Part print with two shaded views. Sizes in mm from the minimum x, y, z corner. A direction names the side the tool comes from. Coordinates: 2 decimals unless noted, no trailing zeros. Loops run counter-clockwise (first coordinate to the right, second up) from the corner with the lowest first, then second, coordinate; pieces in that order, holes last. Notation, with made-up numbers: (80.25, 83.25) -> (137.25, 83.25) arc R9 cw to (137.25, 100.25) -> close; hole circle Ø2 at (1.25, 13). An arc over 180 degrees is marked (long way). Use one line per item in the form item = value.
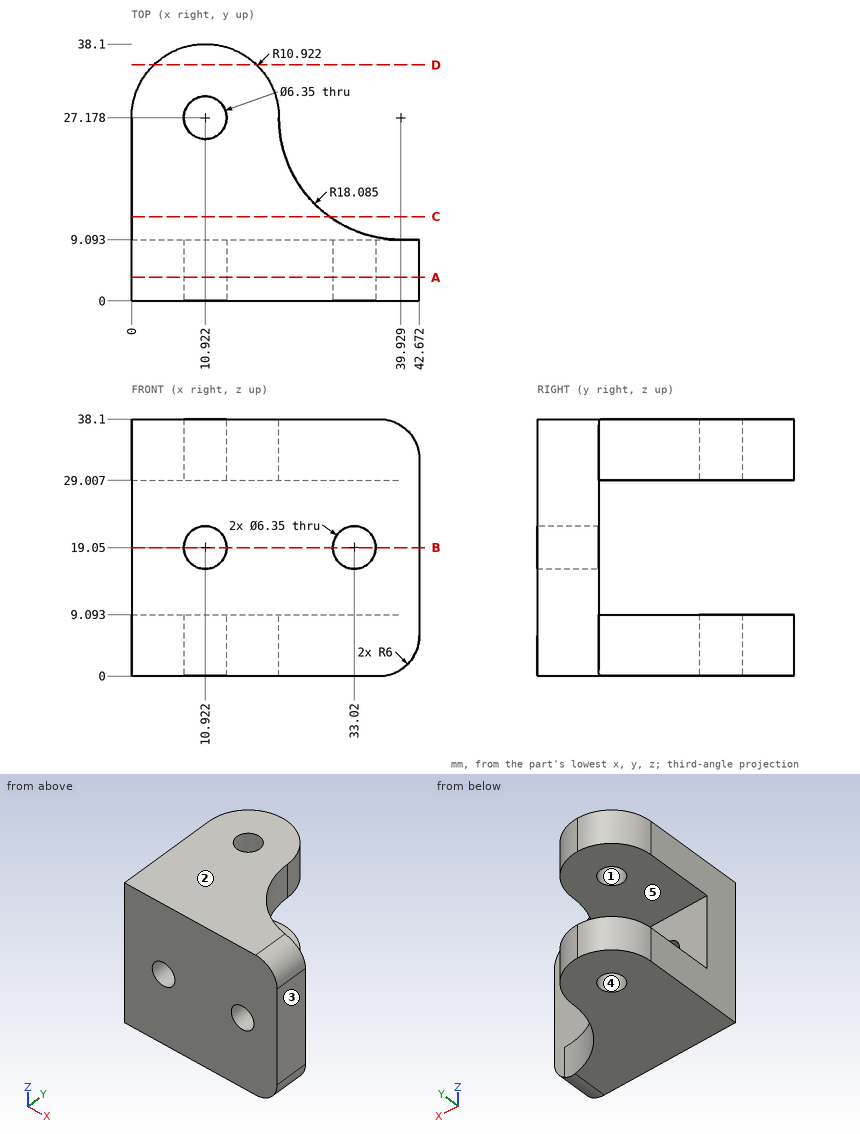
Q1. Which spindle directions (+Z, -Z, +X, -X, +Y, -Y) get a long thin tool onto all of the face, cutting with end or side? Do the marked faces 4 and 5. Say none if no direction does.
Result:
face_4 = +Z, -Z
face_5 = +X, -X, +Y
Q2. Band-saw the part on D-D, the plane y = 35. Write the cut outline in (x, z) (1 decimal), and give its area (3 significant figures).
Result:
outline = (3.3, 0) -> (18.5, 0) -> (18.5, 9.1) -> (3.3, 9.1) -> close; (3.3, 29) -> (18.5, 29) -> (18.5, 38.1) -> (3.3, 38.1) -> close
area = 277 mm2
Q3. Band-saw the part on C-C, the plane y = 12.5. Write the cut outline in (x, z), and give its area (3 significant figures).
Result:
outline = (0, 0) -> (29.36, 0) -> (29.36, 9.09) -> (0, 9.09) -> close; (0, 29.01) -> (29.36, 29.01) -> (29.36, 38.1) -> (0, 38.1) -> close
area = 534 mm2
Q4. Mould opens along X. For the marked faces 1, 2 and 3 say: released by +X, released by -X, zero draft, split by the parting line, or undercut.
Result:
face_1 = undercut
face_2 = zero draft
face_3 = released by +X
Q5. Wall check: line 1 along X through (y, z) = (5.25, 19.05) (3 decimals); line 2 along Z through (x, y) = (19.5, 31); line 3 along Y through (x, z) = (39.5, 3.5). Give the ranges that are in metal, low to high.
Result:
line_1 = 0 to 7.747, 14.097 to 29.845, 36.195 to 42.672
line_2 = 0 to 9.09, 29.01 to 38.1
line_3 = 0 to 9.1
Q6. Pin check, flat tip, straight feed: pin 1 Ø1 at (x, z) = (11, 17) entering from +Y. Stop position of the tip, or through.
Result:
pin_1 = through
Q7. Band-saw the part on B-B, the plane z = 19.05. Write the cut outline in (x, y) (1 decimal).
Result:
outline = (0, 0) -> (7.7, 0) -> (7.7, 9.1) -> (0, 9.1) -> close; (14.1, 0) -> (29.8, 0) -> (29.8, 9.1) -> (14.1, 9.1) -> close; (36.2, 0) -> (42.7, 0) -> (42.7, 9.1) -> (36.2, 9.1) -> close
Q8. Band-saw the part on A-A, the plane y = 3.5. Write the cut outline in (x, z) (3 decimals).
Result:
outline = (0, 0) -> (36.672, 0) arc R6 ccw to (42.672, 6) -> (42.672, 32.1) arc R6 ccw to (36.672, 38.1) -> (0, 38.1) -> close; hole circle Ø6.35 at (10.922, 19.05); hole circle Ø6.35 at (33.02, 19.05)
